from build123d import *

# Parameters (mm, degrees)
SKETCH1_R               = 4.5
BOSS_EXTRUDE1_DEPTH     = 120
BOSS_EXTRUDE2_DEPTH     = 20
CHAMFER1_SIZE           = 1
CUT_EXTRUDE1_DEPTH      = 5.5
CUT_EXTRUDE1_DEPTH_BACK = 5.5


with BuildPart() as part:
    # Sketch1 → Boss-Extrude1 (new body)
    with BuildSketch(Plane(origin=(0, 0, 0), x_dir=(1, 0, 0), z_dir=(0, 1, 0))):
        Circle(SKETCH1_R)
    extrude(amount=BOSS_EXTRUDE1_DEPTH)

    # Sketch2 → Boss-Extrude2 (add)
    with BuildSketch(Plane(origin=(0, 120, 0), x_dir=(1, 0, 0), z_dir=(0, 1, 0))):
        Polygon((1.732050808, 3), (-1.732050808, 3), (-3.464101615, 0), (-1.732050808, -3), (1.732050808, -3), (3.464101615, 0), align=None)
    extrude(amount=BOSS_EXTRUDE2_DEPTH)

    # Chamfer1
    chamfer1_edges = [part.edges().sort_by_distance(p)[0] for p in [
        (-4.5, 120, 0),
    ]]
    chamfer(chamfer1_edges, length=CHAMFER1_SIZE)

    # Sketch3 → Cut-Extrude1 (cut, two sides)
    with BuildSketch(Plane.XY) as cut_extrude1_sk:
        with BuildLine():
            Line((0.75, 0), (2.229044758, 21.151325457))
            ThreePointArc((2.229044758, 21.151325457), (2.910634909, 23.343484317), (4.5, 25))
            Line((4.5, 25), (4.5, 0))
            Line((4.5, 0), (0.75, 0))
        make_face()
        with BuildLine():
            Line((-4.5, 25), (-4.5, 0))
            Line((-4.5, 0), (-0.75, 0))
            Line((-0.75, 0), (-2.229044758, 21.151325457))
            ThreePointArc((-2.229044758, 21.151325457), (-2.910634909, 23.343484317), (-4.5, 25))
        make_face()
    extrude(amount=CUT_EXTRUDE1_DEPTH, mode=Mode.SUBTRACT)
    extrude(cut_extrude1_sk.sketch, amount=-CUT_EXTRUDE1_DEPTH_BACK, mode=Mode.SUBTRACT)


solid = part.part
Can you work these out from the model? Positions are in its coordinate system, mm. A direction names the side the tool comes from. Round coordinates to 2 decimals unless told otherwise and drop trailing zeros. Write each loop counter-clockwise with the first axis right and the second up, starting at its lowest first coordinate (ties: lowest second). Pieces come first, ordered by that corner, then holes. Notation, with made-up numbers: M 64.5,48.25 L 103.5,48.25 A5 cw 103.5,53.25 Z; hole C 40.5,44.5 d10. An arc over 180 degrees is marked long. Use a Markdown table: item, result.
Item 1: Which directions (+Z, -Z, +X, -X, +Y, -Y) give clear straight access to the entire face, cutting with the end or side of a thin tool? Please do faces 1 (the face through (-2.6, 129.9, -1.5)), 2 (the face through (-2.6, 129.9, 1.5)), 3 (the face through (2.6, 129.9, -1.5)), 4 (the face through (0, 130, 3)).
Found:
| item | result |
|---|---|
| face 1 | -Z, -X, +Y |
| face 2 | +Z, -X, +Y |
| face 3 | -Z, +X, +Y |
| face 4 | +Z, +X, -X, +Y |
Item 2: I want a section at B-B (y = 130.5). List the corners of the cut face in (x, z) for me, and give its area (3 significant figures).
Found:
| item | result |
|---|---|
| outline | M -3.46,0 L -1.73,-3 L 1.73,-3 L 3.46,0 L 1.73,3 L -1.73,3 Z |
| area | 31.2 mm2 |
Item 3: If I drill on line 1 along Z through (x, y) = (-0.25, 114); line 2 along Z through (x, y) = (-1.5, 82); line 3 along X through (y, z) = (87, -2), over which ranges is the centre line in solid material (lowest first)? Write a range as [from, to].
Found:
| item | result |
|---|---|
| line 1 | z = [-4.49, 4.49] |
| line 2 | z = [-4.24, 4.24] |
| line 3 | x = [-4.03, 4.03] |
Item 4: I want a section at C-C (y = 18). List the corners of the cut face in (x, z) for me, and give its area (3 significant figures).
Found:
| item | result |
|---|---|
| outline | M -2.01,-4.03 A4.5 ccw 2.01,-4.03 L 2.01,4.03 A4.5 ccw -2.01,4.03 Z |
| area | 34.9 mm2 |
Item 5: I want a section at A-A (y = 37). List the corners of the cut face in (x, z) for me, and give its area (3 significant figures).
Found:
| item | result |
|---|---|
| outline | C 0,0 d9 |
| area | 63.6 mm2 |
Item 6: For pin 1 Ø3 at (x, y) = (0.5, 125) entering from -Z; pin 2 Ø3 at (y, z) = (117, -3) entering from +X; pin 3 Ø3 at (x, y) = (0, 127.5) entering from +Z, each with a flat end and sliding along its axis, tell me the tip position at first contact or that it passes through.
Found:
| item | result |
|---|---|
| pin 1 | stops at z = -3 |
| pin 2 | stops at x = 4.24 |
| pin 3 | stops at z = 3 |
